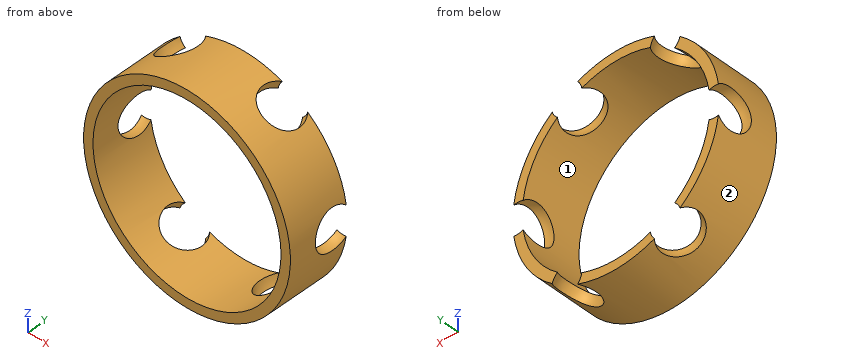
```python
from build123d import *
from build123d.topology import SkipClean

# Parameters (mm, degrees)
SKETCH3_W          = 1
SKETCH3_H          = 10
CIRPATTERN1_COUNT  = 6
SKETCH5_R          = 11
SKETCH5_R_2        = 10
CUT_EXTRUDE1_DEPTH = 3.5


with BuildPart() as part:
    # Sketch3 → Revolve3 (revolve)
    with BuildSketch(Plane.XY, mode=Mode.PRIVATE) as revolve3_sk:
        with Locations((10.5, 0)):
            Rectangle(SKETCH3_W, SKETCH3_H)
    revolve(revolve3_sk.sketch.rotate(Axis((0, 0, 0), (0, 1, 0)), 90), axis=Axis((0, 0, 0), (0, 1, 0)))

    # Sketch4 → Cut-Revolve1 (revolve, cut)
    with SkipClean():  # the faces are left unmerged after this step: merging them gives an invalid solid
        with BuildSketch(Plane.XY, mode=Mode.PRIVATE) as cut_revolve1_sk:
            with BuildLine():
                ThreePointArc((10.5, 2.2), (8.3, 0), (10.5, -2.2))
                Line((10.5, -2.2), (10.5, 2.2))
            make_face()
            with BuildLine():
                Line((10.5, 2.2), (10.5, -2.2))
                ThreePointArc((10.5, -2.2), (12.055634919, -1.555634919), (12.7, 0))
                ThreePointArc((12.7, 0), (12.055634919, 1.555634919), (10.5, 2.2))
            make_face()
        cut_revolve1 = revolve(cut_revolve1_sk.sketch.rotate(Axis((10.5, -2.2, 0), (0, 1, 0)), 264.14281938), axis=Axis((10.5, -2.2, 0), (0, 1, 0)), mode=Mode.SUBTRACT)
    add(part.part.scale(1), mode=Mode.REPLACE)  # the faces are merged on a copy

    # CirPattern1: Cut-Revolve1 ×6 about axis
    cirpattern1_axis = Axis((0, 0, 0), (0, 1, 0))
    for i in range(1, CIRPATTERN1_COUNT):
        add(cut_revolve1.rotate(cirpattern1_axis, i * 360 / CIRPATTERN1_COUNT), mode=Mode.SUBTRACT)

    # Sketch5 → Cut-Extrude1 (cut)
    with BuildSketch(Plane(origin=(0, 5, 0), x_dir=(1, 0, 0), z_dir=(0, 1, 0))):
        with Locations(Location((0, 0, 0), (0, 0, 90))):
            Circle(SKETCH5_R)
        with Locations(Location((0, 0, 0), (0, 0, 90))):
            Circle(SKETCH5_R_2, mode=Mode.SUBTRACT)
    extrude(amount=-CUT_EXTRUDE1_DEPTH, mode=Mode.SUBTRACT)


solid = part.part
```
Input: part model. Units: mm. Frame: model coordinates. Face numbers are marked on the shaded views. Round coordinates to 2 decimals unless told otherwise and drop trailing zeros. Loops run counter-clockwise (first coordinate to the right, second up) from the corner with the lowest first, then second, coordinate; pieces in that order, holes last. Notation, with made-up numbers: (-14, 58.5) -> (8, 58.5) arc R21 cw to (8, 67.5) -> close; hole circle Ø7 at (-34.5, 75). An arc over 180 degrees is marked (long way). Use one line per item in the form item = value. Start each with the question number.
Item 1: Section query B-B on z = -5.25. Return the cut outline in (x, y).
Item 2: Mould query, pull axis Z, two halves, no side actions, for the marked faces 1 and 2. Classes: pulls with the +Z half, pulls with the -Z half, needs draft (parallel to the pull), parting line crosses it, or undercut.
Item 3: Contact query for flat-ended pins moving along their axis: pin 1 Ø1.5 at (x, y) = (-5.5, -3.5) entering from -Z; pin 2 Ø12 at (x, z) = (0, 0) entering from -Y; pin 3 Ø1 at (y, z) = (-3, -7) entering from +X. Output: stop coordinate, or through.
Item 4: Section query C-C on y = -1.25. Return the cut outline in (x, z), then the cut area to 3 significant figures.
Item 5: Section query A-A on x = 0. Return the cut outline in (y, z), then the cut area to 3 significant figures.
Item 6: Material intervals for L1, parallel to X at y = -3.5, z = 0; L2, parallel to Z at x = -4.5, y = -3.5; L3, parallel to X at y = -3, z = 5, sorted ascending. Write a range as from..to.
Item 7: Section query D-D on y = -4.25. Return the cut outline in (x, z).
Ans:
q1.outline = (-9.67, -5) -> (-8.51, -5) -> (-8.51, 1.5) -> (-9.67, 1.5) -> close; (8.51, -5) -> (9.67, -5) -> (9.67, 1.5) -> (8.51, 1.5) -> close
q2.face_1 = undercut
q2.face_2 = parting line crosses it
q3.pin_1 = -9.92
q3.pin_2 = through
q3.pin_3 = 8.87
q4.outline = (-10.86, -1.78) arc R11 ccw to (-6.97, -8.51) arc R1.81 cw to (-6.39, -7.69) arc R10 cw to (-9.86, -1.69) arc R1.81 cw to start; (-10.86, 1.78) arc R1.81 cw to (-9.86, 1.69) arc R10 cw to (-6.39, 7.69) arc R1.81 cw to (-6.97, 8.51) arc R11 ccw to start; (-3.89, -10.29) arc R11 ccw to (3.89, -10.29) arc R1.81 cw to (3.46, -9.38) arc R10 cw to (-3.46, -9.38) arc R1.81 cw to start; (-3.89, 10.29) arc R1.81 cw to (-3.46, 9.38) arc R10 cw to (3.46, 9.38) arc R1.81 cw to (3.89, 10.29) arc R11 ccw to start; (6.39, -7.69) arc R1.81 cw to (6.97, -8.51) arc R11 ccw to (10.86, -1.78) arc R1.81 cw to (9.86, -1.69) arc R10 cw to start; (6.39, 7.69) arc R10 cw to (9.86, 1.69) arc R1.81 cw to (10.86, 1.78) arc R11 ccw to (6.97, 8.51) arc R1.81 cw to start
q4.area = 44.5 mm^2
q5.outline = (-5, -11) -> (1.5, -11) -> (1.5, -10) -> (-5, -10) -> close; (-5, 10) -> (1.5, 10) -> (1.5, 11) -> (-5, 11) -> close
q5.area = 13.0 mm^2
q6.L1 = -11..-10, 10..11
q6.L2 = -10.04..-8.93, 8.93..10.04
q6.L3 = -9.8..-8.66, 8.66..9.8
q7.outline = circle Ø22 at (0, 0); hole circle Ø20 at (0, 0)
